Could you check a few things on this model? Use its own coordinates, in mm. Face numbers are marked on the shaded views. Round coordinates to 2 decimals unless told otherwise and drop trailing zeros. Write each loop counter-clockwise with the first axis right and the second up, starting at its lowest first coordinate (ties: lowest second). Pieces come first, ordered by that corner, then holes. Notation, with made-up numbers: (-10, 72) - (14, 72) arc R30 ccw to (14, 98) - close; hole circle Ø7 at (81, 65.25). An arc over 180 degrees is marked (long way). Write each question's results on one line, items separated by ' | '. Start each with the question number.
(1) Imagine slicing it at C-C on x = 0. Write out the boundary of the cut face in (y, z), then the cut area to 3 significant figures.
(2) Imagine slicing it at B-B on z = 0. Write out the boundary of the cut face in (x, y).
(3) Imagine slicing it at D-D on z = 31. State how many separate pieces and enclosed holes the cut face has, then the cut area to 3 significant figures.
(4) Thinking about a two-plate mould opening in X: for the marked faces 1, 2, 3 and 4, which applies, +X half, -X half, draft (parallel to the pull), parting line (faces both ways), or undercut?
(5) Please list where these lines run through material, in increasing order: line 1 (X direction, y = 5.75, z = 30.75); line 2 (X direction, y = 9.5, z = 0); line 3 (Z direction, x = -13, y = 4). Write a range as [from, to].
(6) Imagine slicing it at A-A on y = 10.5. Write out the boundary of the cut face in (x, z).
```python
from build123d import *

# Parameters (mm, degrees)
SKETCH_1_W      = 70
SKETCH_1_H      = 70
SKETCH_1_R      = 2
SKETCH_1_R_2    = 34
EXTRUDE_1_DEPTH = 15.1
FILLET_1_R      = 5
FILLET_2_R      = 2


with BuildPart() as part:
    # Эскиз1 → Бобышка-Вытянуть1 (new body)
    with BuildSketch(Plane(origin=(0, 0, 0), x_dir=(1, 0, 0), z_dir=(0, 1, 0))):
        Rectangle(SKETCH_1_W, SKETCH_1_H)
        with Locations(Location((30.75, 30.75, 0), (0, 0, 270))):
            Circle(SKETCH_1_R, mode=Mode.SUBTRACT)
        with Locations(Location((0, 0, 0), (0, 0, 270))):
            Circle(SKETCH_1_R_2, mode=Mode.SUBTRACT)
        with Locations(Location((30.75, -30.75, 0), (0, 0, 270))):
            Circle(SKETCH_1_R, mode=Mode.SUBTRACT)
        with Locations(Location((-30.75, -30.75, 0), (0, 0, 270))):
            Circle(SKETCH_1_R, mode=Mode.SUBTRACT)
        with Locations(Location((-30.75, 30.75, 0), (0, 0, 270))):
            Circle(SKETCH_1_R, mode=Mode.SUBTRACT)
    extrude(amount=EXTRUDE_1_DEPTH)

    # Скругление1
    fillet_1_edges = [part.edges().sort_by_distance(p)[0] for p in [
        (35, 7.55, 35),
        (-35, 7.55, 35),
        (-35, 7.55, -35),
        (35, 7.55, -35),
    ]]
    fillet(fillet_1_edges, radius=FILLET_1_R)

    # Скругление2
    # the kernel refuses this fillet: 2 mm, written as the material it takes off along each edge
    with BuildSketch(Plane(origin=(0, 0, 0), x_dir=(0, 0, 1), z_dir=(-1, 0, 0))) as fillet_2_piece_1:
        with BuildLine():
            CenterArc((34 + FILLET_2_R, FILLET_2_R), FILLET_2_R, 180, 90)
            Line((34, FILLET_2_R), (34, 0))
            Line((34, 0), (34 + FILLET_2_R, 0))
        make_face()
    revolve(axis=Axis((0, 0, 0), (0, 1, 0)), mode=Mode.SUBTRACT)
    with BuildSketch(Plane(origin=(0, 15.1, 0), x_dir=(0, 0, 1), z_dir=(-1, 0, 0))) as fillet_2_piece_2:
        with BuildLine():
            CenterArc((34 + FILLET_2_R, -FILLET_2_R), FILLET_2_R, 90, 90)
            Line((34, -FILLET_2_R), (34, 0))
            Line((34, 0), (34 + FILLET_2_R, 0))
        make_face()
    revolve(axis=Axis((0, 15.1, 0), (0, 1, 0)), mode=Mode.SUBTRACT)


solid = part.part
```
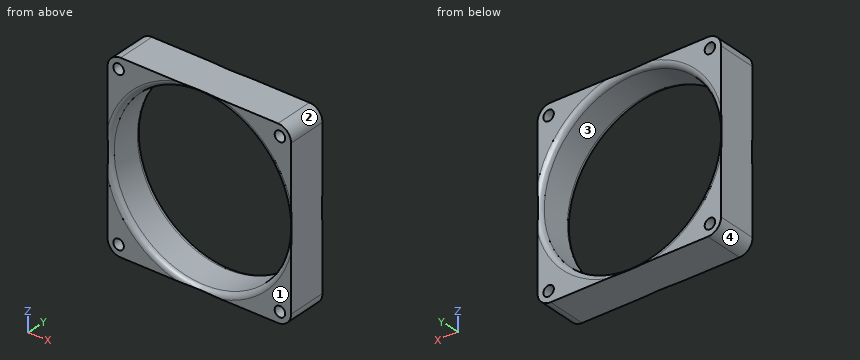
Response:
1) outline: (0.27, -35) - (14.83, -35) arc R2 ccw to (13.1, -34) - (2, -34) arc R2 ccw to start; (0.27, 35) arc R2 ccw to (2, 34) - (13.1, 34) arc R2 ccw to (14.83, 35) - close | area: 27.1 mm²
2) outline: (-35, 0.27) arc R2 ccw to (-34, 2) - (-34, 13.1) arc R2 ccw to (-35, 14.83) - close; (34, 2) arc R2 ccw to (35, 0.27) - (35, 14.83) arc R2 ccw to (34, 13.1) - close
3) separate pieces: 4 | enclosed holes: 0 | area: 504 mm²
4) face 1: draft | face 2: +X half | face 3: undercut | face 4: -X half
5) line 1: [-34.94, -32.75], [-28.75, -14.51], [14.51, 28.75], [32.75, 34.94] | line 2: [-35, -34], [34, 35] | line 3: [-35, -31.42], [31.42, 35]
6) outline: (-35, -30) arc R5 ccw to (-30, -35) - (30, -35) arc R5 ccw to (35, -30) - (35, 30) arc R5 ccw to (30, 35) - (-30, 35) arc R5 ccw to (-35, 30) - close; hole circle Ø68 at (0, 0); hole circle Ø4 at (-30.75, -30.75); hole circle Ø4 at (-30.75, 30.75); hole circle Ø4 at (30.75, -30.75); hole circle Ø4 at (30.75, 30.75)
